Geometry check sheet. Reference: the model listing, model coordinates, mm. Coordinates: 2 decimals unless noted, no trailing zeros. Loops run counter-clockwise (first coordinate to the right, second up) from the corner with the lowest first, then second, coordinate; pieces in that order, holes last.
from build123d import *

# Parameters (mm, degrees)
PAD003_DEPTH           = 3
SKETCH005_W            = 10
SKETCH005_H            = 3
POCKET001_DEPTH        = 3
LINEARPATTERN001_COUNT = 3
LINEARPATTERN001_PITCH = 180


with BuildPart() as part:
    # Sketch004 → Pad003 (new body)
    with BuildSketch(Plane.YZ):
        Polygon((394, 0), (0, 0), (0, -3), (-3, -3), (-3, -13), (0, -13), (0, -16), (394, -16), (394, -13), (397, -13), (397, -3), (394, -3), align=None)
    extrude(amount=PAD003_DEPTH)

    # Sketch005 → Pocket001 (cut)
    with BuildSketch(Plane.YZ.offset(3)):
        with Locations((17, -14.5)):
            Rectangle(SKETCH005_W, SKETCH005_H)
    pocket001 = extrude(amount=-POCKET001_DEPTH, mode=Mode.SUBTRACT)

    # LinearPattern001: Pocket001 ×3
    with Locations(*[(0, i * LINEARPATTERN001_PITCH, 0) for i in range(1, LINEARPATTERN001_COUNT)]):
        add(pocket001, mode=Mode.SUBTRACT)


with BuildPart() as part_1:
    # Body003 placement: moved
    add(part.part.moved(Location((0, 0, 29))))


solid = part_1.part
(1) Gauge pin test, flat ends, axial feed: pin 1 Ø0.9 at (x, y) = (1.5, 395) entering from -Z; pin 2 Ø0.9 at (x, y) = (2, -1.5) entering from +Z; pin 3 Ø0.9 at (x, z) = (1.5, 14) entering from -Y. Record the tip position at first contact, or that the pin passes through.
Findings:
pin 1: stops at z = 16
pin 2: stops at z = 26
pin 3: stops at y = 0
(2) Sectioned sample at A-A on x = 1.35. Record the cut outline in (y, z).
Findings:
outline: (-3, 16) - (0, 16) - (0, 13) - (12, 13) - (12, 16) - (22, 16) - (22, 13) - (192, 13) - (192, 16) - (202, 16) - (202, 13) - (372, 13) - (372, 16) - (382, 16) - (382, 13) - (394, 13) - (394, 16) - (397, 16) - (397, 26) - (394, 26) - (394, 29) - (0, 29) - (0, 26) - (-3, 26) - close
(3) Scan lines: L1, parallel to Y at x = 1.2, z = 14; L2, parallel to Y at x = 2.8, z = 26.5; L3, parallel to Z at x = 1.55, y = 194. Record each from-to range of solid material in increasing order.
Findings:
L1: y = 0 to 12, 22 to 192, 202 to 372, 382 to 394
L2: y = 0 to 394
L3: z = 16 to 29
